from build123d import *

# Parameters (mm, degrees)
SKETCH1_R           = 3.175
BOSS_EXTRUDE1_DEPTH = 508
SKETCH2_W           = 25.4
SKETCH2_H           = 12.7
CUT_EXTRUDE1_DEPTH  = 11.922
LPATTERN1_COUNT     = 10
LPATTERN1_PITCH     = 50.8


with BuildPart() as part:
    # Sketch1 → Boss-Extrude1 (new body)
    with BuildSketch(Plane.XY):
        with BuildLine():
            Line((5.461, 0), (5.461, -38.1))
            Line((5.461, -38.1), (3.175, -38.1))
            Line((3.175, -38.1), (3.175, -4.443185344))
            ThreePointArc((3.175, -4.443185344), (-4.855985791, 2.498384078), (5.461, 0))
        make_face()
        Circle(SKETCH1_R, mode=Mode.SUBTRACT)
    extrude(amount=BOSS_EXTRUDE1_DEPTH)

    # Sketch2 → Cut-Extrude1 (cut, through all)
    with BuildSketch(Plane(origin=(5.461, 0, 0), x_dir=(0, 0, -1), z_dir=(1, 0, 0))):
        with Locations((-495.3, -0.889)):
            Rectangle(SKETCH2_W, SKETCH2_H)
    cut_extrude1 = extrude(amount=-CUT_EXTRUDE1_DEPTH, mode=Mode.SUBTRACT)

    # LPattern1: Cut-Extrude1 ×10
    with Locations(*[(0, 0, -i * LPATTERN1_PITCH) for i in range(1, LPATTERN1_COUNT)]):
        add(cut_extrude1, mode=Mode.SUBTRACT)


solid = part.part
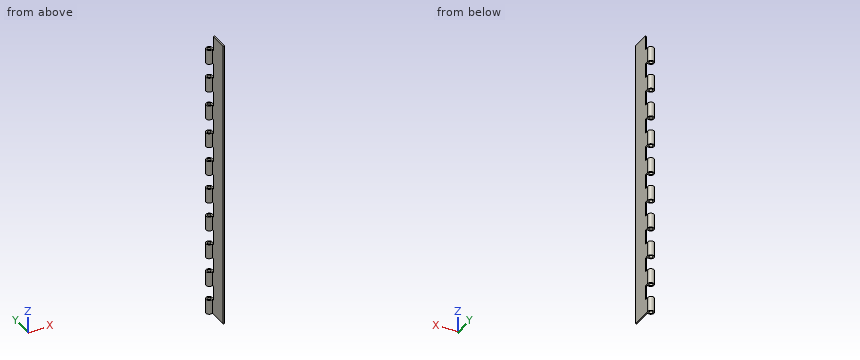
Work out the finished part from the listing and answer in its coordinate system (mm). Round coordinates to 2 decimals unless told otherwise and drop trailing zeros. Order: outer loops, then holes, each group sorted by start corner. A loop starts at its lowest first (then second) coordinate and runs counter-clockwise, first axis right, second up. Notation, with made-up numbers: M 9,13 L 18,13 A23 ccw 18,51 Z; hole C 82,20 d2. An arc over 180 degrees is marked long. Put each result on its own line as item: value. Start each with the question number.
Q1. Section D-D, the plane z = 38 is taken. Write down the section's boundary in (x, y) (3 decimals).
Q2. Section C-C, the plane y = -34 is taken. Write down the section's boundary in (x, z) (3 decimals), and give its area (3 significant figures).
Q3. Flat-ended cylindrical pins translate along their axes: pin 1 (1.5 mm diameter, centred on x = -0.5, z = 125, fed in from -Y); pin 2 (1.1 mm diameter, centred on x = 4, z = 498.5, fed in from +Y); pin 3 (4 mm diameter, centred on x = 0, y = 0, fed in from -Z); pin 4 (3.5 mm diameter, centred on x = -1.5, y = -3.5, fed in from -Z). Find the tip coordinate at first contact, or state that the pin passes through.
Q4. Straight lines are drawn through the part: L1, parallel to Y at x = -0.75, z = 169.5; L2, parallel to Y at x = 0, z = 370.25 (3 decimals); L3, parallel to Y at x = 4.25, z = 332. For each, find the intervals that lie inside material, in ascending order. Write a range as [from, to].
Q5. Section B-B, the plane x = 0 is taken. Give the number of separate pieces and of enclosed holes in the cut face, and give its area (3 significant figures).
Q6. Section A-A, the plane z = 316 is taken. Write down the section's boundary in (x, y) (3 decimals).
Findings below:
1. outline: M 3.175,-38.1 L 5.461,-38.1 L 5.461,-7.239 L 3.175,-7.239 Z
2. outline: M 3.175,0 L 5.461,0 L 5.461,508 L 3.175,508 Z
2. area: 1,160 mm^2
3. pin 1: stops at y = -5.46
3. pin 2: stops at y = -7.24
3. pin 3: passes through
3. pin 4: stops at z = 0
4. L1: y = [-5.41, -3.09], [3.09, 5.41]
4. L2: y = [-5.461, -3.175], [3.175, 5.461]
4. L3: y = [-38.1, -7.24]
5. separate pieces: 20
5. enclosed holes: 0
5. area: 1,160 mm^2
6. outline: M 3.175,-38.1 L 5.461,-38.1 L 5.461,0 A5.461 ccw long 3.175,-4.443 Z; hole C 0,0 d6.35
